```python
from build123d import *

# Parameters (mm, degrees)
SKETCH2_R           = 3.95
BOSS_EXTRUDE1_DEPTH = 10
BOSS_EXTRUDE1_TAPER = 5


with BuildPart() as part:
    # Sketch1 → Revolve1 (revolve)
    with BuildSketch(Plane.XY):
        with BuildLine():
            Line((0, 3.95), (0, -3.95))
            ThreePointArc((0, -3.95), (3.95, 0), (0, 3.95))
        make_face()
    revolve(axis=Axis((0, 3.95, 0), (0, -1, 0)))

    # Sketch2 → Boss-Extrude1 (add)
    with BuildSketch(Plane.XY):
        Circle(SKETCH2_R)
    extrude(amount=BOSS_EXTRUDE1_DEPTH, taper=BOSS_EXTRUDE1_TAPER)

    # Sketch3 → Revolve2 (revolve)
    with BuildSketch(Plane.XY.offset(10)):
        with BuildLine():
            Line((0, 3.075113365), (0, -3.075113365))
            ThreePointArc((0, -3.075113365), (3.075113365, 0), (0, 3.075113365))
        make_face()
    revolve(axis=Axis((0, 3.075113365, 10), (0, -1, 0)))


solid = part.part
```
Can you work these out from the model? Positions are in its coordinate system, mm. Round coordinates to 2 decimals unless told otherwise and drop trailing zeros. Loops run counter-clockwise (first coordinate to the right, second up) from the corner with the lowest first, then second, coordinate; pieces in that order, holes last. Notation, with made-up numbers: M 8.5,26.5 L 18.5,26.5 A25 ccw 18.5,46.5 Z; hole C 33,42 d1. An arc over 180 degrees is marked long. Answer as a JSON object with one key per item and string values. Group by question number.
Q1. Imagine slicing it at A-A, the plane x = 0. Please give me the cut outline in (y, z), then the cut area to 3 significant figures.
Q2. Imagine slicing it at C-C, the plane z = 11.75. Please give me the cut outline in (x, y), then the cut area to 3 significant figures.
Q3. Please list where these lines run through material, in increasing order: L1, parallel to Z at x = 0, y = 0; L2, parallel to Z at x = 2, y = -1.25; L3, parallel to Y at x = 0, z = 5.5.
Q4. Imagine slicing it at D-D, the plane z = 8.25. Please give me the cut outline in (x, y).
Q5. Will these pins go through, and if not, where does the flat tip stop? pin 1 (1 mm diameter, centred on x = 0.5, y = -2.5, fed in from +Z); pin 2 (2 mm diameter, centred on y = -2.5, z = -2, fed in from +X); pin 3 (4 mm diameter, centred on x = -2, y = -0.5, fed in from +Z); pin 4 (3 mm diameter, centred on x = -2.5, y = 0.5, fed in from -Z).
Findings:
{
 "1": {"outline": "M -3.89,0.69 A3.95 ccw long 3.89,0.69 L 3.08,10 A3.08 ccw -3.08,10 Z", "area": "110 mm2"},
 "2": {"outline": "C 0,0 d5.06", "area": "20.1 mm2"},
 "3": {"L1": "z = -3.95 to 13.08", "L2": "z = -3.17 to 11.97", "L3": "y = -3.47 to 3.47"},
 "4": {"outline": "C 0,0 d6.46"},
 "5": {"pin 1": "stops at z = 12.29", "pin 2": "stops at x = 3.28", "pin 3": "stops at z = 13.07", "pin 4": "stops at z = -3.81"}
}
